from build123d import *

# Parameters (mm, degrees)
F0_R     = 6.096
F1_DEPTH = 16.9164
F2_R     = 9.525
F2_R_2   = 6.096
F3_DEPTH = 3.175
F4_R     = 9.525
F5_DEPTH = 3.175


# Not quite as in the source:
# - a feature names something its author has since deleted; it is built from what else it names


with BuildPart() as f1:
    # F0 (on Top) → F1 (new body)
    with BuildSketch(Plane.XY):
        Circle(F0_R)
    extrude(amount=F1_DEPTH)

    # F2 (on face) → F3 (join)
    with BuildSketch(Plane.XY.offset(16.9164)):
        Circle(F2_R)
        Circle(F2_R_2, mode=Mode.SUBTRACT)
        Circle(F2_R_2)
    extrude(amount=F3_DEPTH)

    # F4 (on face) → F5 (join)
    with BuildSketch(Plane(origin=(0, 0, 0), x_dir=(1, 0, 0), z_dir=(0, 0, -1))):
        Circle(F4_R)
    extrude(amount=F5_DEPTH)


solid = f1.part
The model under review builds one solid part; all positions refer to its coordinate system, in mm. A direction names the side the tool comes from. Coordinates: 2 decimals unless noted, no trailing zeros. Write each loop counter-clockwise with the first axis right and the second up, starting at its lowest first coordinate (ties: lowest second). Pieces come first, ordered by that corner, then holes. Notation, with made-up numbers: M -39,19.5 L 7,19.5 A24 cw 7,29.5 Z; hole C -5.75,-34 d9. An arc over 180 degrees is marked long. Put each result on its own line as item: value.
1) Add section C-C on z = 13.5. Give the boundary of the cut face in (x, y).
Computed:
outline: C 0,0 d12.19
2) Add section A-A on x = 0. Give the boundary of the cut face in (y, z) (3 decimals).
Computed:
outline: M -9.525,-3.175 L 9.525,-3.175 L 9.525,0 L 6.096,0 L 6.096,16.916 L 9.525,16.916 L 9.525,20.091 L -9.525,20.091 L -9.525,16.916 L -6.096,16.916 L -6.096,0 L -9.525,0 Z
3) For faces 5 (the flat face through (2, -6, 16.916)), 6 (the cylindrical face through (-7.559, 5.796, -1.565)), list the 3-axis set-ups (+Z, -Z, +X, -X, +Y, -Y) from which the entire face can be reached by the end or side of a thin tool; tool diameter is ignored.
Computed:
face 5: none
face 6: +Z, -Z
4) Wall thickness on probe 1 along Z at (x, y) = (-6.25, -5.25) (3 decimals); probe 2 along X at (y, z) = (2.75, 12.25); probe 3 along X at (y, z) = (8.25, -2): over which ranges is each line inside the solid? List them lowest first. Write a range as [from, to].
Computed:
probe 1: z = [-3.175, 0], [16.916, 20.091]
probe 2: x = [-5.44, 5.44]
probe 3: x = [-4.76, 4.76]
5) Draft analysis for pull direction Z (two halves, no side actions). For faces 1 (the flat face through (0, 0, 20.091)), 2 (the flat face through (0, 0, -3.175)), 3 (the cylindrical face through (-0.794, 6.044, 8.34)), 4 (the cylindrical face through (-7.559, -5.796, 18.482)), state which applies: released by +Z, released by -Z, zero draft, split by the parting line, or undercut.
Computed:
face 1: released by +Z
face 2: released by -Z
face 3: undercut
face 4: zero draft
6) Clearance check with flat-ended pins moving along their axes: pin 1 Ø8 at (y, z) = (-5, 8.5) entering from -X; pin 2 Ø2 at (x, z) = (3.5, 13) entering from +Y; pin 3 Ø6 at (y, z) = (1, 8) entering from -X. State where each tip first meets the part, or that it passes through.
Computed:
pin 1: stops at x = -6.01
pin 2: stops at y = 5.56
pin 3: stops at x = -6.1
